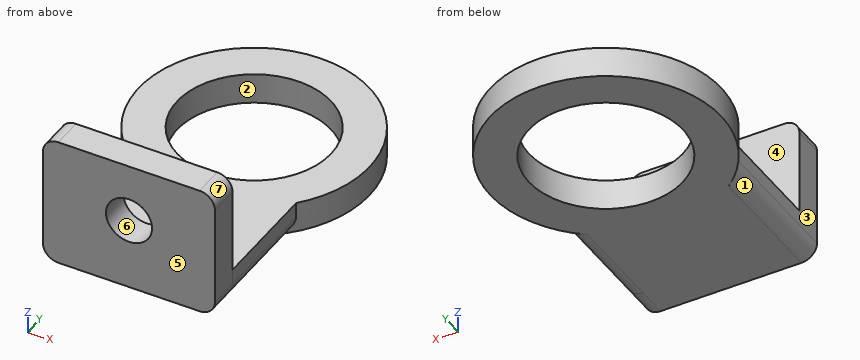
Autodesk Inventor part; units mm, degrees
ref_plane "YZ Plane" through (0, 0, 0) normal (1, 0, 0) x (0, 1, 0)
ref_plane "XZ Plane" through (0, 0, 0) normal (0, 1, 0) x (-1, 0, 0)
ref_plane "XY Plane" through (0, 0, 0) normal (0, 0, 1) x (1, 0, 0)
sketch "Sketch1" plane through (0, 0, 0) normal (0, 0, 1) x (1, 0, 0)
  circle A0 centre (0, 0) radius 4.85
  circle A1 centre (0, 0) radius 5
  circle A2 centre (0, 0) radius 7.5
  dimension "d0" = 10
  dimension "d1" = 15
extrude "Extrusion1" add sketch "Sketch1" along normal mid plane 2 contours A2
sketch "Sketch2" plane through (0, 0, 1) normal (0, 0, 1) x (1, 0, 0)
  circle A0 centre (0, 0) radius 7.5
  line L0 (-5.5902, -5) -> (0, -5)
  line L1 (0, -5) -> (0, -7.5)
  line L2 (-5.5902, -7.5) -> (-5.5902, -5)
  circle A1 centre (0, 0) radius 7.5
  line L3 (5.5902, -5) -> (0, -5)
  line L4 (5.5902, -7.5) -> (5.5902, -5)
  line L5 (3.3913, -9.725) -> (-18.205, -9.725)
  line L6 (-5.5902, -7.5) -> (-5.5902, -9.725)
  line L7 (5.5902, -9.725) -> (5.5902, -7.5)
  line L8 (5.5902, -9.725) -> (5.5902, -12.225)
  line L9 (5.5902, -12.225) -> (-5.5902, -12.225)
  line L10 (-5.5902, -12.225) -> (-5.5902, -9.725)
  dimension "d13" = 2.5
extrude "Extrusion2" add sketch "Sketch2" against normal blind 2 contours A0 L4 L7 L8 L9 L10 L6 L2 | A0 L1 L3
sketch "Sketch5" plane through (-5.5902, -12.225, 1) normal (0, -1, 0) x (1, 0, 0)
  line L0 (11.1803, -2) -> (11.1803, 6.5)
  line L1 (11.1803, 6.5) -> (0, 6.5)
  line L2 (0, 6.5) -> (0, -2)
  line L3 (0, -2) -> (11.1803, -2)
  line L4 (11.1803, -2) -> (11.1803, 6.5)
  point P0 (5.5902, -1)
  dimension "d14" = 8.5
extrude "Extrusion5" add sketch "Sketch5" along normal blind 2
sketch "Sketch6" plane through (-5.5902, -14.225, 1) normal (0, -1, 0) x (1, 0, 0)
  line L0 (11.1803, 6.5) -> (0, 6.5)
  line L1 (5.5902, 6.5) -> (5.5902, 2.69)
  circle A0 centre (5.5902, 2.69) radius 1.5
  point P0 (5.5902, -1)
  dimension "d17" = 3.81
  dimension "d18" = 3
extrude "Extrusion6" cut sketch "Sketch6" against normal blind 2
fillet "Fillet1" radius 1 4 edges at (5.5902, -13.225, 7.5) (-5.5902, -13.225, 7.5) (5.5902, -9.6125, -1) (-5.5902, -9.6125, -1)
properties part number "SyringeTailConnector"
Design review of the part built by this model. Coordinates are the model's own, in mm. Face numbers are marked on the shaded views. A direction names the side the tool comes from. Give positions to 0.01 mm unless a question says otherwise; leave off trailing zeros. Write each loop counter-clockwise with the first axis right and the second up, starting at its lowest first coordinate (ties: lowest second). Pieces come first, ordered by that corner, then holes. Notation, with made-up numbers: (6.25, -28) - (61.25, -28) arc R9 cw to (61.25, -20) - close; hole circle Ø10 at (37.5, 40.5). An arc over 180 degrees is marked (long way). Return JSON: item names as keys, results as strings. Group by question number.
(1) Mouldability with a two-part tool opening along X and no side actions: class the marked faces 5, 6 and 7 as +X half, -X half, draft (parallel to the pull), parting line (faces both ways), or undercut.
(2) Machinability: for the marked faces 1, 2, 3 and 4, which of the approach directions +Z, -Z, +X, -X, +Y, -Y give a long, thin tool a straight path to every point of the face, cutting with its end or side? Answer none if there is none.
(3) We need section B-B, the plane x = 0. Give the boundary of the cut face in (y, z) (3 decimals), then the cut area to 4 significant figures.
(4) Insertion check: pin 1 (1.5 mm diameter, centred on x = 4.5, y = 4.5, fed in from +Z); pin 2 (2 mm diameter, centred on y = -2, z = 0.5, fed in from +X); pin 3 (0.8 mm diameter, centred on y = -7, z = 0.5, fed in from +X). Each pin has a flat end and moves straight along its axis. Give the tip position at first contact, or say it passes through.
(5) We need section A-A, the plane y = 0. Give the boundary of the cut face in (x, z).
(6) To check wall thickness, follow probe 1 along Y at (x, z) = (0, 0.05) (3 decimals); probe 2 along X at (y, z) = (-13.35, 3.69); probe 3 along Z at (x, y) = (3.75, -11.5). State the ranges of each line that lie inside material, in increasing order.
(7) We need section D-D, the plane x = 4.25. Give the boundary of the cut face in (y, z) (3 decimals).
(8) We need section C-C, the plane z = 3.69. Give the boundary of the cut face in (x, y) (3 decimals).
Reported:
{
 "1": {"face 5": "draft", "face 6": "undercut", "face 7": "+X half"},
 "2": {"face 1": "-Z, -X, -Y", "face 2": "+Z, -Z", "face 3": "+Z, -Z, -X, -Y", "face 4": "+Z, +X, -X, +Y"},
 "3": {"outline": "(-14.225, -1) - (-5, -1) - (-5, 1) - (-12.225, 1) - (-12.225, 2.19) - (-14.225, 2.19) - close; (-14.225, 5.19) - (-12.225, 5.19) - (-12.225, 7.5) - (-14.225, 7.5) - close; (5, -1) - (7.5, -1) - (7.5, 1) - (5, 1) - close", "area": "30.45 mm2"},
 "4": {"pin 1": "stops at z = 1", "pin 2": "stops at x = 7.43", "pin 3": "stops at x = 5.59"},
 "5": {"outline": "(-7.5, -1) - (-5, -1) - (-5, 1) - (-7.5, 1) - close; (5, -1) - (7.5, -1) - (7.5, 1) - (5, 1) - close"},
 "6": {"probe 1": "y = -14.225 to -5, 5 to 7.5", "probe 2": "x = -5.59 to -1.5, 1.5 to 5.59", "probe 3": "z = -1 to 1"},
 "7": {"outline": "(-14.225, -1) - (-2.634, -1) - (-2.634, 1) - (-12.225, 1) - (-12.225, 7.5) - (-14.225, 7.5) - close; (2.634, -1) - (6.18, -1) - (6.18, 1) - (2.634, 1) - close"},
 "8": {"outline": "(-5.59, -14.225) - (-1.5, -14.225) - (-1.5, -12.225) - (-5.59, -12.225) - close; (1.5, -14.225) - (5.59, -14.225) - (5.59, -12.225) - (1.5, -12.225) - close"}
}
